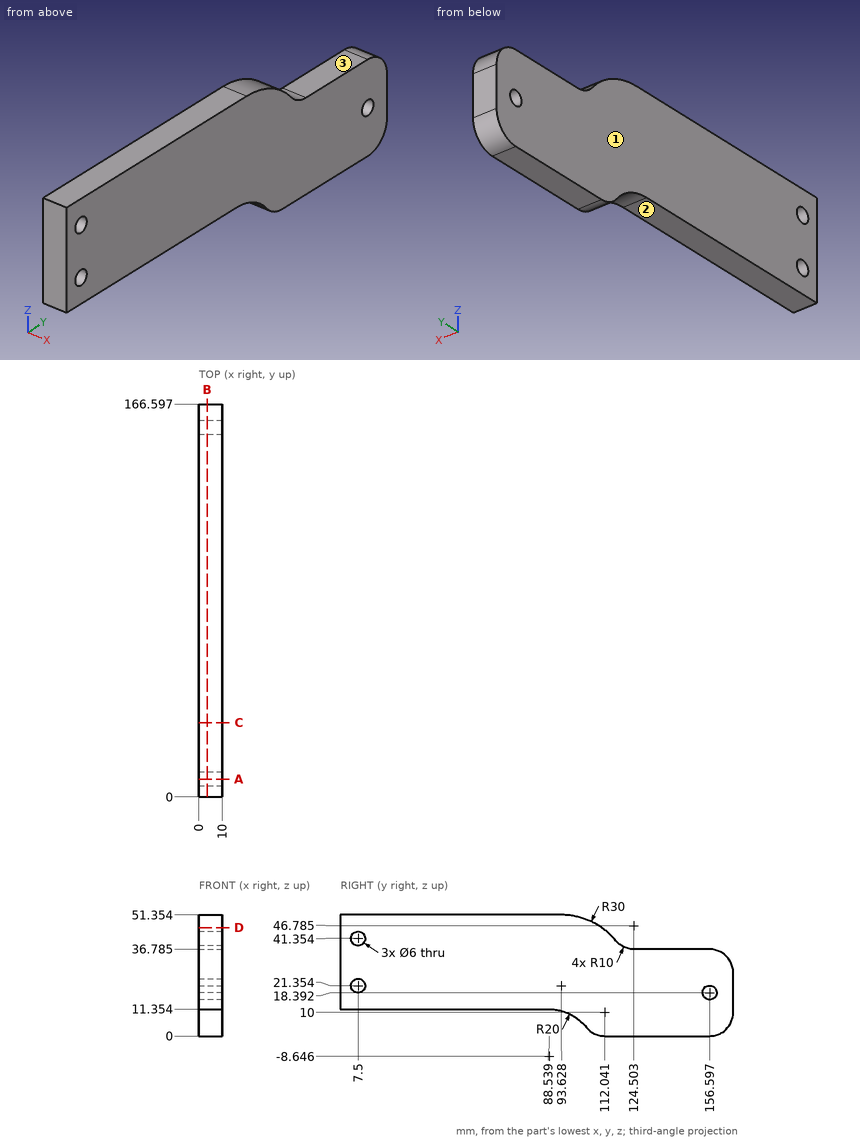
Source: three-view drawing plus pictorial views. Frame: mm from the lowest corner of the part. A direction names the side the tool comes from. Coordinates: 2 decimals unless noted, no trailing zeros. Order: outer loops, then holes, each group sorted by start corner. A loop starts at its lowest first (then second) coordinate and runs counter-clockwise, first axis right, second up. Notation, with made-up numbers: M 35.25,-7 L 39.25,-7 A31 ccw 39.25,18 Z; hole C 9.5,84.25 d6. An arc over 180 degrees is marked long. One line per question, with ' | ' between items. Start each with the question number.
Item 1: Ray query, probe 1 along Z at (x, y) = (9.25, 125) (1 decimal); probe 2 along Z at (x, y) = (1.5, 46); probe 3 along Y at (x, z) = (2.5, 20) (1 decimal). Return the intervals inside material, ascending. Write a range as [from, to].
Item 2: Pin query (flat end, axial travel): pin 1 Ø3 at (x, y) = (7, 143) entering from +Z (1 decimal); pin 2 Ø3 at (x, y) = (4, 27) entering from -Z. Return the tip coordinate at first contact, or that it passes through.
Item 3: Cut plane C-C, the plane y = 31.5. Return the cut outline in (x, z).
Item 4: Set-up query: the marked faces 1, 2 and 3. Return all of +Z, -Z, +X, -X, +Y, -Y with unobstructed straight access to the full face (end or side cutting, diameter ignored); none if empty.
Item 5: Cut plane B-B, the plane x = 3.5. Return the cut outline in (y, z) (1 decimal).
Item 6: Cut plane A-A, the plane y = 7.5. Return the cut outline in (x, z).
Item 7: Cut plane D-D, the plane z = 46. Return the cut outline in (x, y).
A:
1) probe 1: z = [0, 36.8] | probe 2: z = [11.35, 51.35] | probe 3: y = [0, 4.8], [10.2, 154.1], [159.1, 166.6]
2) pin 1: stops at z = 36.8 | pin 2: stops at z = 11.35
3) outline: M 0,11.35 L 10,11.35 L 10,51.35 L 0,51.35 Z
4) face 1: +Z, -Z, -X, +Y, -Y | face 2: -Z, +X, -X, -Y | face 3: +Z, +X, -X, +Y
5) outline: M 0,11.4 L 88.5,11.4 A20 cw 104.2,3.8 A10 ccw 112,0 L 156.6,0 A10 ccw 166.6,10 L 166.6,26.8 A10 ccw 156.6,36.8 L 124.5,36.8 A10 cw 116.8,40.4 A30 ccw 93.6,51.4 L 0,51.4 Z; hole C 7.5,21.4 d6; hole C 7.5,41.4 d6; hole C 156.6,18.4 d6
6) outline: M 0,11.35 L 10,11.35 L 10,18.35 L 0,18.35 Z; M 0,24.35 L 10,24.35 L 10,38.35 L 0,38.35 Z; M 0,44.35 L 10,44.35 L 10,51.35 L 0,51.35 Z
7) outline: M 0,0 L 10,0 L 10,110.73 L 0,110.73 Z
